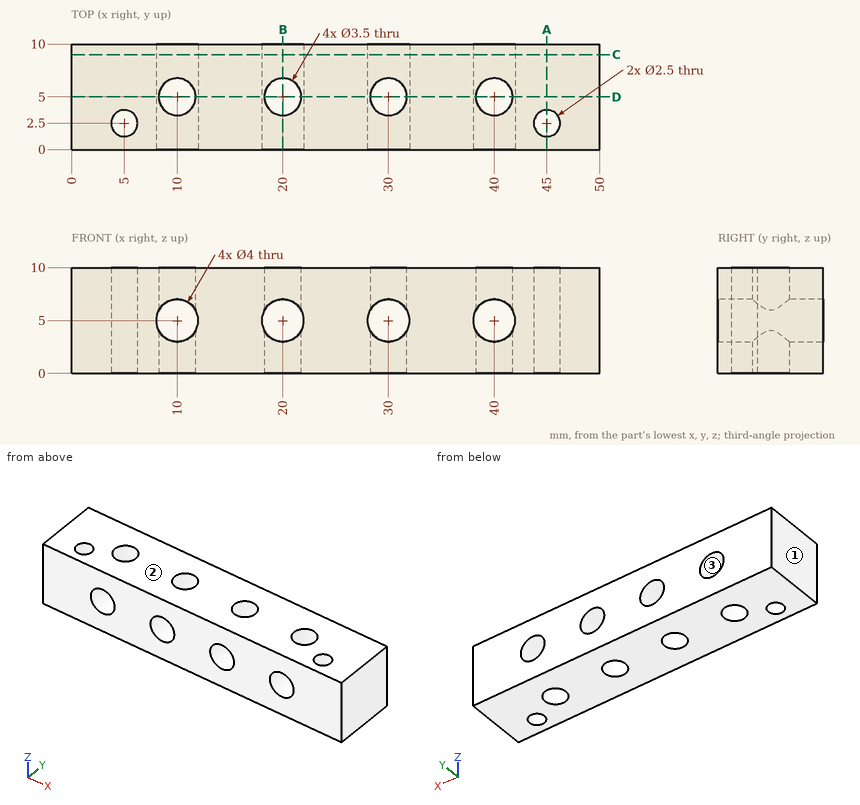
Geometry check sheet. Reference: drawing and pictorial views, mm from the part's lowest x, y, z. Round coordinates to 2 decimals unless told otherwise and drop trailing zeros. Loops run counter-clockwise (first coordinate to the right, second up) from the corner with the lowest first, then second, coordinate; pieces in that order, holes last. Notation, with made-up numbers: (-28, -33.75) -> (17, -33.75) arc R32 cw to (17, 1.25) -> close; hole circle Ø3 at (-1, 39.25). An arc over 180 degrees is marked (long way). Answer as a JSON object with one key per item and string values.
Q1. Section check C-C (y = 9). Record the boundary of the cut face in (x, z).
Data:
{"outline": "(0, 0) -> (50, 0) -> (50, 10) -> (0, 10) -> close; hole circle Ø4 at (10, 5); hole circle Ø4 at (20, 5); hole circle Ø4 at (30, 5); hole circle Ø4 at (40, 5)"}
Q2. Draft check along Z on the marked faces 1, 2 and 3. Enter one of: pulls with the +Z half, pulls with the -Z half, needs draft (parallel to the pull), parting line crosses it, or undercut.
Data:
{"face 1": "needs draft", "face 2": "pulls with the +Z half", "face 3": "undercut"}
Q3. Section check B-B (x = 20). Record the boundary of the cut face in (y, z).
Data:
{"outline": "(0, 0) -> (3.25, 0) -> (3.25, 3) -> (0, 3) -> close; (0, 7) -> (3.25, 7) -> (3.25, 10) -> (0, 10) -> close; (6.75, 0) -> (10, 0) -> (10, 3) -> (6.75, 3) -> close; (6.75, 7) -> (10, 7) -> (10, 10) -> (6.75, 10) -> close"}
Q4. Section check A-A (x = 45). Record the boundary of the cut face in (y, z), then the cut area to 3 significant figures.
Data:
{"outline": "(0, 0) -> (1.25, 0) -> (1.25, 10) -> (0, 10) -> close; (3.75, 0) -> (10, 0) -> (10, 10) -> (3.75, 10) -> close", "area": "75.0 mm2"}
Q5. Section check D-D (y = 5). State how many separate pieces and enclosed holes the cut face has, then the cut area to 3 significant figures.
Data:
{"separate pieces": "5", "enclosed holes": "0", "area": "357 mm2"}
Q6. Scan lines: line 1 (X direction, y = 4.5, z = 5); line 2 (X direction, y = 1, z = 3.75); line 3 (X direction, y = 1.5, z = 0.75). Record each from-to range of solid material in increasing order. Write a range as from..to.
Data:
{"line 1": "x = 0..8, 12..18, 22..28, 32..38, 42..50", "line 2": "x = 0..8.44, 11.56..18.44, 21.56..28.44, 31.56..38.44, 41.56..50", "line 3": "x = 0..4.25, 5.75..44.25, 45.75..50"}
